Design review of the part shown in the three views and the two pictorial views. Dimensions are in mm from the part's minimum x, y and z. A direction names the side the tool comes from. Coordinates: 2 decimals unless noted, no trailing zeros. Loops run counter-clockwise (first coordinate to the right, second up) from the corner with the lowest first, then second, coordinate; pieces in that order, holes last. Notation, with made-up numbers: (10, 25) - (44, 25) arc R14 cw to (44, 29) - close; hole circle Ø2 at (43.5, 76). An arc over 180 degrees is marked (long way). One line per item, written item: value. Start each with the question number.
1. Take a section at C-C, the plane z = 11. State the section outline as (x, y) points, and give its area (3 significant figures).
2. Insertion check: pin 1 (12 mm diameter, centred on x = 106.5, z = 51.5, fed in from +Y). The pin has a flat end and moves straight along its axis. Give the tip position at first contact, or say it passes through.
3. To check wall thickness, follow line 1 (Z direction, x = 19, y = 10); line 2 (Y direction, x = 84.5, z = 64). State the ranges of each line that lie inside material, in increasing order. Write a range as from..to.
4. For the marked faces 1 and 2, list the 3-axis set-ups (+Z, -Z, +X, -X, +Y, -Y) from which the entire face can be reached by the end or side of a thin tool; tool diameter is ignored.
5. The part is to be moulded in two halves that separate along X. For the marked faces 3, 4, 5 and 6, say which applies: released by +X, released by -X, zero draft, split by the parting line, or undercut.
6. Take a section at A-A, the plane y = 24. State the section outline as (x, z) points, and give its area (3 significant figures).
7. Take a section at B-B, the plane x = 83. State the section outline as (y, z) points.
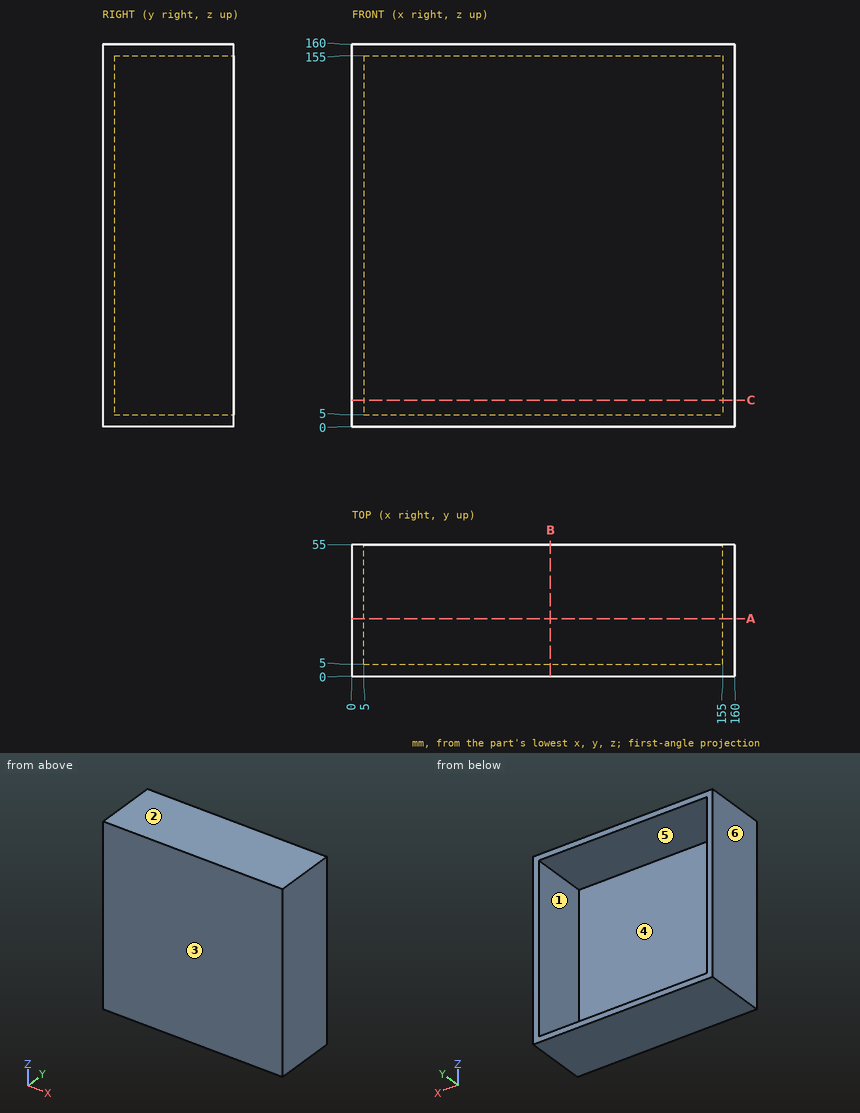
Solutions:
1. outline: (0, 0) - (160, 0) - (160, 55) - (155, 55) - (155, 5) - (5, 5) - (5, 55) - (0, 55) - close
1. area: 1,300 mm2
2. pin 1: y = 5
3. line 1: 0..5, 155..160
3. line 2: 0..5
4. face 1: +Y
4. face 2: +Z, +X, -X, +Y, -Y
5. face 3: zero draft
5. face 4: undercut
5. face 5: undercut
5. face 6: released by -X
6. outline: (0, 0) - (160, 0) - (160, 160) - (0, 160) - close; hole (5, 5) - (155, 5) - (155, 155) - (5, 155) - close
6. area: 3,100 mm2
7. outline: (0, 0) - (55, 0) - (55, 5) - (5, 5) - (5, 155) - (55, 155) - (55, 160) - (0, 160) - close
